```python
from build123d import *

# Parameters (mm, degrees)
BOSS_EXTRUDE1_DEPTH = 8.9


with BuildPart() as part:
    # Sketch1 → Boss-Extrude1 (new body)
    with BuildSketch(Plane(origin=(0, 0, 0), x_dir=(1, 0, 0), z_dir=(0, 1, 0))):
        with BuildLine():
            Line((0, -26.575), (130.828205579, -26.575))
            ThreePointArc((130.828205579, -26.575), (132.830371988, -13.354485299), (133.5, 0))
            ThreePointArc((133.5, 0), (132.830371988, 13.354485299), (130.828205579, 26.575))
            Line((130.828205579, 26.575), (0, 26.575))
            ThreePointArc((0, 26.575), (26.575, 0), (0, -26.575))
        make_face()
    extrude(amount=BOSS_EXTRUDE1_DEPTH)


solid = part.part
```
Source: CAD feature listing. Evaluate the final solid. Frame: model axes, mm. Round coordinates to 2 decimals unless told otherwise and drop trailing zeros. Order: outer loops, then holes, each group sorted by start corner. A loop starts at its lowest first (then second) coordinate and runs counter-clockwise, first axis right, second up. Notation, with made-up numbers: (18, 12) -> (66, 12) arc R27 ccw to (66, 40) -> close; hole circle Ø7 at (88.5, 88.5). An arc over 180 degrees is marked (long way). One line per item, written item: value. Start each with the question number.
Q1. Section query D-D (z = -9.5). Return the cut outline in (x, y).
Q2. Section query A-A (x = 18). Return the cut outline in (y, z) (3 decimals).
Q3. Section query B-B (y = 5.25). Return the cut outline in (x, z) (3 decimals).
Q4. Section query C-C (z = 13.5). Return the cut outline in (x, y), plus the area to 3 significant figures.
Q5. Material intervals for probe 1 along Z at (x, y) = (7, 2.5) (1 decimal); probe 2 along Z at (x, y) = (22, 2.25) (3 decimals); probe 3 along X at (y, z) = (5.25, 1), sorted ascending.
Q6. Pin query (flat end, axial travel): pin 1 (5 mm diameter, centred on y = 1, z = 17, fed in from +X); pin 2 (5 mm diameter, centred on y = 3.5, z = -12.5, fed in from +X); pin 3 (3 mm diameter, centred on y = 2.5, z = -8.5, fed in from -X). Return the tip coordinate at first contact, or that it passes through.
Findings below:
1. outline: (24.82, 0) -> (133.16, 0) -> (133.16, 8.9) -> (24.82, 8.9) -> close
2. outline: (0, -26.575) -> (8.9, -26.575) -> (8.9, -19.551) -> (0, -19.551) -> close; (0, 19.551) -> (8.9, 19.551) -> (8.9, 26.575) -> (0, 26.575) -> close
3. outline: (0, -26.575) -> (130.828, -26.575) arc R133.5 ccw to (130.828, 26.575) -> (0, 26.575) arc R26.575 cw to start
4. outline: (22.89, 0) -> (132.82, 0) -> (132.82, 8.9) -> (22.89, 8.9) -> close
4. area: 978 mm²
5. probe 1: -26.6 to -25.6, 25.6 to 26.6
5. probe 2: -26.575 to -14.907, 14.907 to 26.575
5. probe 3: 26.56 to 133.5
6. pin 1: x = 132.71
6. pin 2: x = 133.12
6. pin 3: x = 24.62
